Part print with two shaded views. Sizes in mm from the minimum x, y, z corner. Round coordinates to 2 decimals unless told otherwise and drop trailing zeros. Write each loop counter-clockwise with the first axis right and the second up, starting at its lowest first coordinate (ties: lowest second). Pieces come first, ordered by that corner, then holes. Notation, with made-up numbers: (5.25, 25) -> (62.25, 25) arc R9 cw to (62.25, 39) -> close; hole circle Ø2 at (85, -15.75). An arc over 180 degrees is marked (long way). Return JSON: item names as keys, results as strings. Group by question number.
(1) Drill centre lines: L1, parallel to Y at x = 25.5, z = 0.8; L2, parallel to X at y = 28.5, z = 2.6 (1 decimal); L3, parallel to Y at x = 18, z = 1.1 (1 decimal). Where is each one in solid material? Low to high. Write a range as from..to.
(2) Drop a flat-ended pin along its axis: pin 1 Ø2 at (x, y) = (25.63, 36.85) entering from -Z. Give the stop position or say it passes through.
(3) Saw through at D-D (y = 50). List the corners of the cut face in (x, z) (1 decimal).
(4) Saw through at B-B (z = 1.2). List the corners of the cut face in (x, y) (1 decimal).
(5) Saw through at C-C (x = 5). List the corners of the cut face in (y, z) (1 decimal).
(6) Saw through at A-A (y = 34). List the corners of the cut face in (x, z) (1 decimal), plus the area to 3 significant figures.
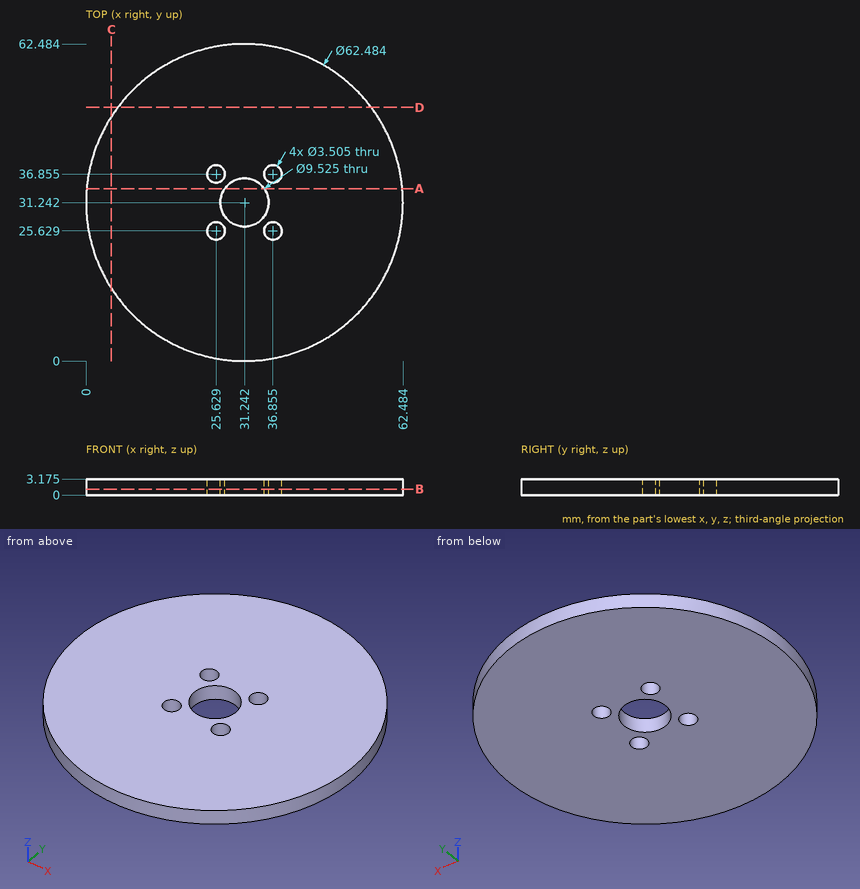
Computed values:
{
 "1": {"L1": "0.53..23.88, 27.38..35.11, 38.6..61.95", "L2": "0.1..27.3, 35.1..62.4", "L3": "2.9..59.5"},
 "2": {"pin 1": "through"},
 "3": {"outline": "(6.3, 0) -> (56.2, 0) -> (56.2, 3.2) -> (6.3, 3.2) -> close"},
 "4": {"outline": "circle Ø62.5 at (31.2, 31.2); hole circle Ø3.5 at (25.6, 25.6); hole circle Ø3.5 at (25.6, 36.9); hole circle Ø9.5 at (31.2, 31.2); hole circle Ø3.5 at (36.9, 25.6); hole circle Ø3.5 at (36.9, 36.9)"},
 "5": {"outline": "(14.3, 0) -> (48.2, 0) -> (48.2, 3.2) -> (14.3, 3.2) -> close"},
 "6": {"outline": "(0.1, 0) -> (27.4, 0) -> (27.4, 3.2) -> (0.1, 3.2) -> close; (35.1, 0) -> (62.4, 0) -> (62.4, 3.2) -> (35.1, 3.2) -> close", "area": "173 mm2"}
}
